Model file for the job. Use its own axes, mm. Face numbers are marked on the shaded views. A direction names the side the tool comes from. Give positions to 0.01 mm unless a question says otherwise; leave off trailing zeros. Loops run counter-clockwise (first coordinate to the right, second up) from the corner with the lowest first, then second, coordinate; pieces in that order, holes last. Notation, with made-up numbers: M -3,84.5 L 34,84.5 A22 cw 34,94.5 Z; hole C 18.25,-38 d7. An arc over 180 degrees is marked long. Answer in a Markdown table with one row per item.
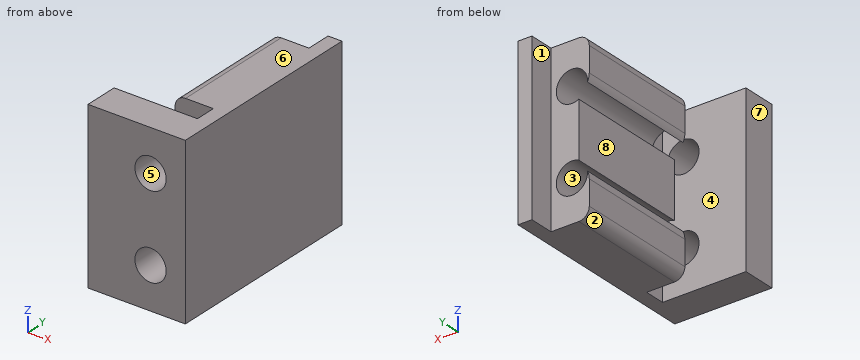
```python
from build123d import *

# Parameters (mm, degrees)
SKETCH1_W           = 12
SKETCH1_H           = 24
BOSS_EXTRUDE1_DEPTH = 4.9
SKETCH2_W           = 2
SKETCH2_H           = 24
BOSS_EXTRUDE2_DEPTH = 29.5
BOSS_EXTRUDE4_START = 3
SKETCH4_W           = 5.5
SKETCH4_H           = 24
BOSS_EXTRUDE4_DEPTH = 18
SKETCH5_W           = 9.25
SKETCH5_H           = 18
CUT_EXTRUDE1_DEPTH  = 1.5
FILLET1_R           = 2.5
SKETCH6_R           = 2.25
CUT_EXTRUDE2_DEPTH  = 30.644729717
FILLET2_R           = 1.5


with BuildPart() as part:
    # Sketch1 → Boss-Extrude1 (new body)
    with BuildSketch(Plane(origin=(0, 0, 0), x_dir=(1, 0, 0), z_dir=(0, 1, 0))):
        Rectangle(SKETCH1_W, SKETCH1_H)
    extrude(amount=BOSS_EXTRUDE1_DEPTH)

    # Sketch2 → Boss-Extrude2 (add)
    with BuildSketch(Plane(origin=(0, 0, 0), x_dir=(1, 0, 0), z_dir=(0, 1, 0))):
        with Locations((7, 0)):
            Rectangle(SKETCH2_W, SKETCH2_H)
    extrude(amount=BOSS_EXTRUDE2_DEPTH)

    # Sketch4 → Boss-Extrude4 (add)
    with BuildSketch(Plane(origin=(0, 4.9, 0), x_dir=(1, 0, 0), z_dir=(0, 1, 0)).offset(BOSS_EXTRUDE4_START)):
        with Locations((3.25, 0)):
            Rectangle(SKETCH4_W, SKETCH4_H)
    extrude(amount=BOSS_EXTRUDE4_DEPTH)

    # Sketch5 → Cut-Extrude1 (cut)
    with BuildSketch(Plane.ZY.offset(-0.5)):
        with Locations((0, 16.9)):
            Rectangle(SKETCH5_W, SKETCH5_H)
    extrude(amount=-CUT_EXTRUDE1_DEPTH, mode=Mode.SUBTRACT)

    # Fillet1
    # the kernel refuses this fillet: 2.5 mm, written as the material it takes off along each edge
    with BuildSketch(Plane(origin=(0.5, 31.628219619, 4.625), x_dir=(0, 0, 1), z_dir=(0, -1, 0)), Plane(origin=(0.5, 7.9, -4.625), x_dir=(0, 0, -1), z_dir=(0, 1, 0))) as fillet1_piece_1:
        with BuildLine():
            CenterArc((2.291287847, -2.5), FILLET1_R, 90, 66.421821522)
            Line((0, -1.5), (0, 0))
            Line((0, 0), (2.291287847, 0))
        make_face()
    extrude(amount=23.728219619, mode=Mode.SUBTRACT)

    # Sketch6 → Cut-Extrude2 (cut, through all)
    with BuildSketch(Plane(origin=(0, 25.9, 0), x_dir=(1, 0, 0), z_dir=(0, 1, 0))):
        with Locations(Location((3, -6, 0), (0, 0, 270))):
            Circle(SKETCH6_R)
        with Locations(Location((3, 6, 0), (0, 0, 270))):
            Circle(SKETCH6_R)
    extrude(amount=-CUT_EXTRUDE2_DEPTH, mode=Mode.SUBTRACT)

    # Fillet2
    fillet2_edges = [part.edges().sort_by_distance(p)[0] for p in [
        (0.5, 16.9, -12),
        (0.5, 16.9, 12),
    ]]
    fillet(fillet2_edges, radius=FILLET2_R)


solid = part.part
```
(1) Saw through at C-C, the plane y = 12.75. Give the cut face in (x, z), and give its area (3 significant figures).
Established:
| item | result |
|---|---|
| outline | M 0.5,-10.5 A1.5 ccw 2,-12 L 8,-12 L 8,12 L 2,12 A1.5 ccw 0.5,10.5 L 0.5,6.92 A2.5 ccw 0.76,5.81 A2.25 cw long 2,3.98 L 2,-3.98 A2.25 cw long 0.76,-5.81 A2.5 ccw 0.5,-6.92 Z |
| area | 133 mm2 |
(2) Wall check: L1, parallel to Z at x = 3, y = 20.5; L2, parallel to Z at x = 4.5, y = 24.25; L3, parallel to Y at x = 4, z = -1. Give the ranges that are in metal, low to high.
Established:
| item | result |
|---|---|
| L1 | z = -12 to -8.25, -3.75 to 3.75, 8.25 to 12 |
| L2 | z = -12 to -7.68, -4.32 to 4.32, 7.68 to 12 |
| L3 | y = 0 to 4.9, 7.9 to 25.9 |
(3) Which spindle directions (+Z, -Z, +X, -X, +Y, -Y) get a long thin tool onto all of the face, cutting with end or side? Do the marked faces 1, 2, 3 and 4. Say none if no direction does.
Established:
| item | result |
|---|---|
| face 1 | +Z, -Z, -X, +Y |
| face 2 | -Z, -X, +Y |
| face 3 | +Y, -Y |
| face 4 | +Z, -Z, -X |
(4) Saw through at B-B, the plane z = 1.25. Give the cut face in (x, y).
Established:
| item | result |
|---|---|
| outline | M -6,0 L 8,0 L 8,29.5 L 6,29.5 L 6,25.9 L 2,25.9 L 2,7.9 L 6,7.9 L 6,4.9 L -6,4.9 Z |
(5) Saw through at D-D, the plane x = -0.75. Give the cut face in (y, z), and give its area (3 significant figures).
Established:
| item | result |
|---|---|
| outline | M 0,-12 L 4.9,-12 L 4.9,12 L 0,12 Z |
| area | 118 mm2 |
(6) Mould opens along Z. For the marked faces 5, 6, 7 and 8 say: pulls with the +Z half, pulls with the -Z half, needs draft (parallel to the pull), parting line crosses it, or undercut.
Established:
| item | result |
|---|---|
| face 5 | undercut |
| face 6 | pulls with the +Z half |
| face 7 | needs draft |
| face 8 | undercut |
(7) Flat gauge pins, fed straight in: P1, Ø1.6, axis at x = 3, z = 1.5, coming from the -Y side; P2, Ø4, axis at y = 13.5, z = 0, coming from the -X side; P3, Ø1.8, axis at y = 19, z = -8.5, coming from the -X side; P4, Ø1.1, axis at y = 28.5, z = 6, coming from the -X side. Where does each tip first touch, or does it go through?
Established:
| item | result |
|---|---|
| P1 | stops at y = 0 |
| P2 | stops at x = 2 |
| P3 | stops at x = 0.5 |
| P4 | stops at x = 6 |
(8) Saw through at A-A, the plane x = 3. Give the cut face in (y, z), and give its area (4 significant figures).
Established:
| item | result |
|---|---|
| outline | M 0,-12 L 4.9,-12 L 4.9,-8.25 L 0,-8.25 Z; M 0,-3.75 L 4.9,-3.75 L 4.9,3.75 L 0,3.75 Z; M 0,8.25 L 4.9,8.25 L 4.9,12 L 0,12 Z; M 7.9,-12 L 25.9,-12 L 25.9,-8.25 L 7.9,-8.25 Z; M 7.9,-3.75 L 25.9,-3.75 L 25.9,3.75 L 7.9,3.75 Z; M 7.9,8.25 L 25.9,8.25 L 25.9,12 L 7.9,12 Z |
| area | 343.5 mm2 |
